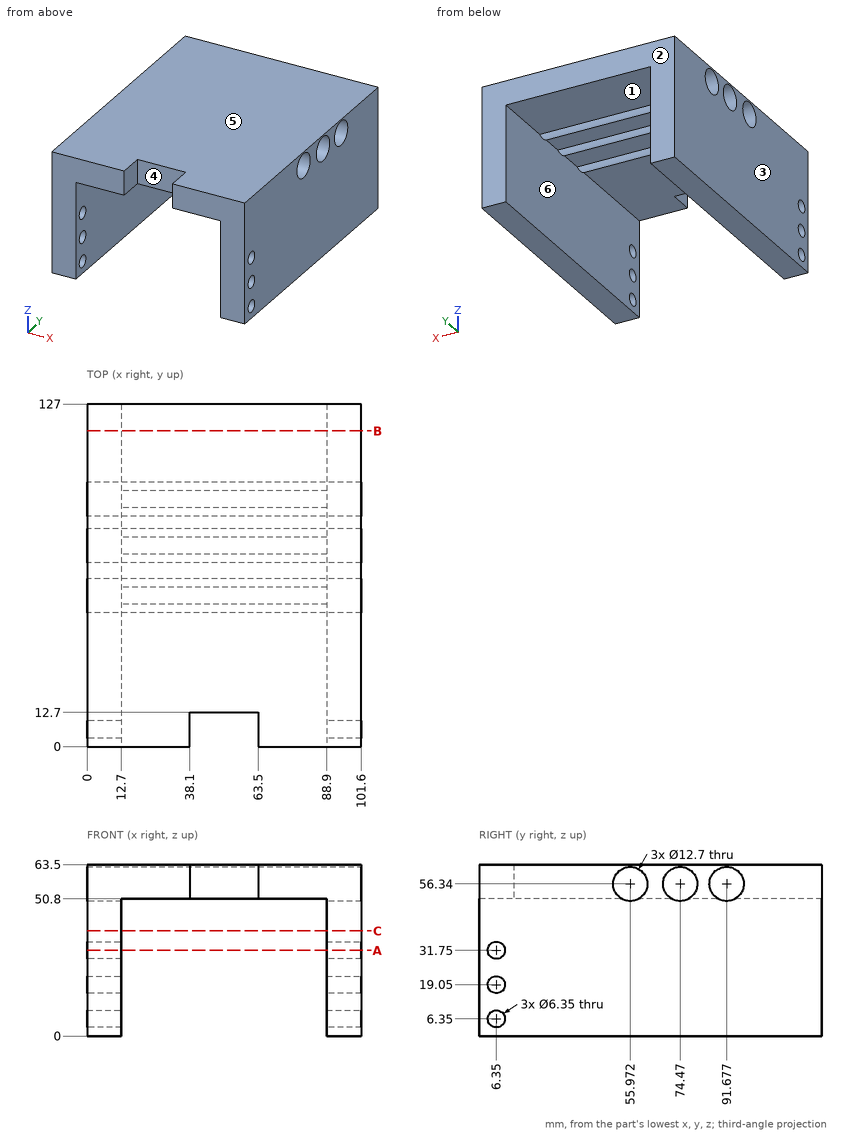
The figure shows three views and two pictorial views of one solid part (mm, origin at its lowest corner). Answer the questions. A direction names the side the tool comes from. Give positions to 0.01 mm unless a question says otherwise; leave off trailing zeros. Write each loop counter-clockwise with the first axis right and the second up, starting at its lowest first coordinate (ties: lowest second). Pieces come first, ordered by that corner, then holes. Notation, with made-up numbers: (40.5, 64) - (62.5, 64) arc R27 cw to (62.5, 103) - close; hole circle Ø6 at (-24, 57.25). An arc over 180 degrees is marked (long way). Return JSON: item names as keys, results as strings.
Q1. Given P1, Ø20.5, axis at y = 91.68, z = 56.34, coming from the -X side; P2, Ø1, axis at x = 19.5, y = 101.5, coming from the -Z side; P3, Ø5, axis at y = 6.35, z = 19.05, coming from the +X side; P4, Ø10, axis at x = 48.5, z = 57.5, coming from the -Y side, each flat-ended and moving along its own axis, determine where each tip first touches the part or whether it passes through.
Reply:
{"P1": "x = 0", "P2": "z = 50.8", "P3": "through", "P4": "y = 12.7"}
Q2. A cutting plane is placed at A-A, the plane z = 31.75. Determine the outline of the cut face in (x, y) (1 decimal).
Reply:
{"outline": "(0, 0) - (12.7, 0) - (12.7, 3.2) - (0, 3.2) - close; (0, 9.5) - (12.7, 9.5) - (12.7, 127) - (0, 127) - close; (88.9, 0) - (101.6, 0) - (101.6, 3.2) - (88.9, 3.2) - close; (88.9, 9.5) - (101.6, 9.5) - (101.6, 127) - (88.9, 127) - close"}
Q3. For the marked faces 4, 5 and 6, determine the directions among +Z, -Z, +X, -X, +Y, -Y from which every point of the face is accessible in a straight line to the end or side of a thin tool.
Reply:
{"face 4": "+Z, -Z, -Y", "face 5": "+Z, +X, -X, +Y, -Y", "face 6": "-Z, +Y, -Y"}
Q4. A cutting plane is placed at B-B, the plane y = 117. Determine the outline of the cut face in (x, z), and give its area (3 significant figures).
Reply:
{"outline": "(0, 0) - (12.7, 0) - (12.7, 50.8) - (88.9, 50.8) - (88.9, 0) - (101.6, 0) - (101.6, 63.5) - (0, 63.5) - close", "area": "2,580 mm²"}
Q5. For a pull along X with two mould halves and no side action, classify the marked faces 1, 2 and 3 as released by +X, released by -X, zero draft, split by the parting line, or undercut.
Reply:
{"face 1": "undercut", "face 2": "zero draft", "face 3": "released by -X"}
Q6. Consider line 1 along Z through (x, y) = (7, 6) (1 decimal); line 2 along X through (y, z) = (58, 40); line 3 along Y through (x, z) = (55, 60). Determine where each line is inside the solid, lowest interval first. Write a range as [from, to].
Reply:
{"line 1": "[0, 3.2], [9.5, 15.9], [22.2, 28.6], [34.9, 63.5]", "line 2": "[0, 12.7], [88.9, 101.6]", "line 3": "[12.7, 50.78], [61.16, 69.28], [79.66, 86.49], [96.87, 127]"}
Q7. A cutting plane is placed at C-C, the plane z = 39. Determine the outline of the cut face in (x, y).
Reply:
{"outline": "(0, 0) - (12.7, 0) - (12.7, 127) - (0, 127) - close; (88.9, 0) - (101.6, 0) - (101.6, 127) - (88.9, 127) - close"}
